For this review, take the finished solid that the model builds, in its own axes (mm). Give positions to 0.01 mm unless a question says otherwise; leave off trailing zeros. Write each loop counter-clockwise with the first axis right and the second up, starting at its lowest first coordinate (ties: lowest second). Pieces come first, ordered by that corner, then holes.
from build123d import *

# Parameters (mm, degrees)
SKETCH1_R           = 1.5
SKETCH1_R_2         = 12
SKETCH1_R_3         = 3
SKETCH1_W           = 2.8
SKETCH1_H           = 30
BOSS_EXTRUDE4_DEPTH = 3


with BuildPart() as part:
    # Sketch1 → Boss-Extrude4 (new body)
    with BuildSketch(Plane(origin=(0, 0, 0), x_dir=(1, 0, 0), z_dir=(0, 1, 0))):
        with BuildLine():
            Line((-121.196449229, -126.808304592), (-11.829794241, -126.808304592))
            ThreePointArc((-11.829794241, -126.808304592), (9.383409194, -118.021508028), (18.170205759, -96.808304592))
            Line((18.170205759, -96.808304592), (18.170205759, -42.124977099))
            ThreePointArc((18.170205759, -42.124977099), (-66.513121735, 42.558350395), (-151.196449229, -42.124977099))
            Line((-151.196449229, -42.124977099), (-151.196449229, -96.808304592))
            ThreePointArc((-151.196449229, -96.808304592), (-142.409652664, -118.021508028), (-121.196449229, -126.808304592))
        make_face()
        with Locations(Location((-19.417066349, 12.133998526, 0), (0, 0, 270))):
            Circle(SKETCH1_R, mode=Mode.SUBTRACT)
        with Locations(Location((-113.609177122, 12.133998526, 0), (0, 0, 270))):
            Circle(SKETCH1_R, mode=Mode.SUBTRACT)
        with Locations(Location((8.170205759, -42.124977099, 0), (0, 0, 270))):
            Circle(SKETCH1_R, mode=Mode.SUBTRACT)
        with Locations(Location((-141.196449229, -42.124977099, 0), (0, 0, 270))):
            Circle(SKETCH1_R, mode=Mode.SUBTRACT)
        with Locations(Location((-66.513121735, 5.435278237, 0), (0, 0, 270))):
            Circle(SKETCH1_R_2, mode=Mode.SUBTRACT)
        with Locations(Location((-66.513121735, 25.558350395, 0), (0, 0, 270))):
            Circle(SKETCH1_R_3, mode=Mode.SUBTRACT)
        with Locations(Location((-66.513121735, -69.564721763, 0), (0, 0, 270))):
            Circle(SKETCH1_R_2, mode=Mode.SUBTRACT)
        with Locations(Location((-123.013121735, -10.138406212, 0), (0, 0, 270))):
            Circle(SKETCH1_R, mode=Mode.SUBTRACT)
        with Locations(Location((-10.013121735, -10.138406212, 0), (0, 0, 270))):
            Circle(SKETCH1_R, mode=Mode.SUBTRACT)
        with Locations(Location((-10.013121735, -121.478406212, 0), (0, 0, 270))):
            Circle(SKETCH1_R, mode=Mode.SUBTRACT)
        with Locations(Location((-123.013121735, -121.478406212, 0), (0, 0, 270))):
            Circle(SKETCH1_R, mode=Mode.SUBTRACT)
        with Locations(Location((-66.513121735, -109.124977099, 0), (0, 0, 270))):
            Circle(SKETCH1_R, mode=Mode.SUBTRACT)
        with Locations(Location((-66.513121735, -24.124977099, 0), (0, 0, 270))):
            Circle(SKETCH1_R, mode=Mode.SUBTRACT)
        with Locations(Location((-141.196449229, -109.124977099, 0), (0, 0, 270))):
            Circle(SKETCH1_R, mode=Mode.SUBTRACT)
        with Locations(Location((8.170205759, -109.124977099, 0), (0, 0, 270))):
            Circle(SKETCH1_R, mode=Mode.SUBTRACT)
        with Locations(Location((-19.417066349, -63.912266725, 0), (0, 0, 270))):
            Circle(SKETCH1_R, mode=Mode.SUBTRACT)
        with Locations(Location((-113.609177122, -63.912266725, 0), (0, 0, 270))):
            Circle(SKETCH1_R, mode=Mode.SUBTRACT)
        with Locations(Location((-85.109177122, 31.058350391, 0), (0, 0, 270))):
            Circle(SKETCH1_R, mode=Mode.SUBTRACT)
        with Locations(Location((-47.917066349, 31.058350391, 0), (0, 0, 270))):
            Circle(SKETCH1_R, mode=Mode.SUBTRACT)
        with Locations((-14.413121735, -25.911649605)):
            Rectangle(SKETCH1_W, SKETCH1_H, mode=Mode.SUBTRACT)
        with Locations((-118.613121735, -25.911649605)):
            Rectangle(SKETCH1_W, SKETCH1_H, mode=Mode.SUBTRACT)
    extrude(amount=BOSS_EXTRUDE4_DEPTH)


solid = part.part
(1) We need section A-A (z = 76). Write out the cut boundary in (x, y).
(2) We need section C-C (z = 33.5). Write out the cut boundary in (x, y).
(3) For L1, parallel to Z at x = -141, y = 0.7; L2, parallel to X at y = 2.5, z = 11; L3, parallel to X at y = 0.9, z = -13, list the stretches that pass through material, from the lowest coordinate up.
(4) We need section B-B (y = 0.6). Count the separate pieces of the cut face and the enclosed holes in it, and give its area (3 significant figures).
(5) Clearance check with flat-ended pins moving along their axes: pin 1 Ø1.5 at (y, z) = (1, 18.5) entering from -X; pin 2 Ø1 at (y, z) = (2.5, 31.5) entering from -X. State where each tip first meets the part, or that it passes through.
(6) We need section D-D (x = -105.5). Write out the cut boundary in (y, z), and give its area (3 significant figures).
(7) The part is to be moulded in two halves that separate along Z. For faces 1 (the cylindrical face through (9.1, 1.5, 118.3)), 2 (the flat face through (-68, 3, 41)), 3 (the cylindrical face through (-69.175, 1.479, -24.174)), say which applies: +Z half, -Z half, draft (parallel to the pull), parting line (faces both ways), or undercut.
The answers:
1. outline: (-151.2, 0) - (-76.64, 0) - (-76.64, 3) - (-151.2, 3) - close; (-56.38, 0) - (18.17, 0) - (18.17, 3) - (-56.38, 3) - close
2. outline: (-150.76, 0) - (-120.01, 0) - (-120.01, 3) - (-150.76, 3) - close; (-117.21, 0) - (-15.81, 0) - (-15.81, 3) - (-117.21, 3) - close; (-13.01, 0) - (17.73, 0) - (17.73, 3) - (-13.01, 3) - close
3. L1: z = 1.84 to 40.64, 43.61 to 107.64, 110.61 to 119.34
3. L2: x = -145.27 to -124.24, -121.79 to -120.01, -117.21 to -15.81, -13.01 to -11.24, -8.79 to 12.24
3. L3: x = -130.8 to -114.83, -112.38 to -75.83, -57.2 to -20.64, -18.19 to -2.23
4. separate pieces: 1
4. enclosed holes: 21
4. area: 24,000 mm2
5. pin 1: stops at x = -148.05
5. pin 2: stops at x = -150.59
6. outline: (0, -33.05) - (3, -33.05) - (3, 126.81) - (0, 126.81) - close
6. area: 480 mm2
7. face 1: +Z half
7. face 2: draft
7. face 3: undercut
